```python
from build123d import *

# Parameters (mm, degrees)
SKETCH_1_R          = 100
EXTRUDE_2_DEPTH     = 50
SHELL_2_T           = -5
SKETCH_6_W          = 41.456951092
SKETCH_6_H          = 6.735302979
CUT_EXTRUDE_1_DEPTH = 10
SKETCH_9_R          = 97
CUT_EXTRUDE_2_DEPTH = 10
SKETCH_13_W         = 6
SKETCH_13_H         = 15.793483952
SKETCH_13_H_2       = 15
CUT_EXTRUDE_3_DEPTH = 10
SKETCH_16_W         = 8.245924623
SKETCH_16_H         = 19.966088532
SKETCH_16_H_2       = 20.04266097
CUT_EXTRUDE_6_DEPTH = 10
SKETCH_17_W         = 4.583098869
SKETCH_17_H         = 14.94320697
SKETCH_17_H_2       = 15.359126099
CUT_EXTRUDE_7_DEPTH = 10
SKETCH_18_W         = 6.507967363
SKETCH_18_H         = 16.40128849
SKETCH_18_H_2       = 16.311833417
CUT_EXTRUDE_8_DEPTH = 10


with BuildPart() as part:
    # Sketch 1 → Extrude 2 (new body)
    with BuildSketch(Plane.XY):
        Circle(SKETCH_1_R)
    extrude(amount=EXTRUDE_2_DEPTH)

    # Shell 2
    shell_2_openings = [part.faces().sort_by_distance(p)[0] for p in [
        (0, 0, 50),
    ]]
    offset(amount=SHELL_2_T, openings=shell_2_openings, kind=Kind.INTERSECTION)

    # Sketch 6 → Cut-Extrude 1 (cut)
    with BuildSketch(Plane.XY):
        with Locations((-20.728475546, 53.011479478)):
            Rectangle(SKETCH_6_W, SKETCH_6_H)
        with Locations((20.728475546, 53.011479478)):
            Rectangle(SKETCH_6_W, SKETCH_6_H)
    extrude(amount=CUT_EXTRUDE_1_DEPTH, mode=Mode.SUBTRACT)

    # Sketch 9 → Cut-Extrude 2 (cut)
    with BuildSketch(Plane.XY.offset(50)):
        Circle(SKETCH_9_R)
    extrude(amount=-CUT_EXTRUDE_2_DEPTH, mode=Mode.SUBTRACT)

    # Sketch 13 → Cut-Extrude 3 (cut)
    with BuildSketch(Plane.ZY.offset(100)):
        with Locations((49.635646507, 7.103258024)):
            Rectangle(SKETCH_13_W, SKETCH_13_H)
        with Locations((49.635646507, -8.293483952)):
            Rectangle(SKETCH_13_W, SKETCH_13_H_2)
    extrude(amount=-CUT_EXTRUDE_3_DEPTH, mode=Mode.SUBTRACT)

    # Sketch 16 → Cut-Extrude 6 (cut)
    with BuildSketch(Plane(origin=(100, 0, 0), x_dir=(0, 0, -1), z_dir=(1, 0, 0))):
        with Locations((-10.841517517, 9.983044266)):
            Rectangle(SKETCH_16_W, SKETCH_16_H)
        with Locations((-10.841517517, -10.021330485)):
            Rectangle(SKETCH_16_W, SKETCH_16_H_2)
    extrude(amount=-CUT_EXTRUDE_6_DEPTH, mode=Mode.SUBTRACT)

    # Sketch 17 → Cut-Extrude 7 (cut)
    with BuildSketch(Plane(origin=(-70.710678119, -70.710678119, 0), x_dir=(0, 0, -1), z_dir=(-0.7071067811865464, -0.7071067811865488, 0))):
        with Locations((-47.581138772, 7.471603485)):
            Rectangle(SKETCH_17_W, SKETCH_17_H)
        with Locations((-47.581138772, -7.67956305)):
            Rectangle(SKETCH_17_W, SKETCH_17_H_2)
    extrude(amount=-CUT_EXTRUDE_7_DEPTH, mode=Mode.SUBTRACT)

    # Sketch 18 → Cut-Extrude 8 (cut)
    with BuildSketch(Plane(origin=(-70.710678119, 70.710678119, 0), x_dir=(0, 0, 1), z_dir=(-0.7071067811865487, 0.7071067811865465, 0))):
        with Locations((49.297240538, 8.200644245)):
            Rectangle(SKETCH_18_W, SKETCH_18_H)
        with Locations((49.297240538, -8.155916709)):
            Rectangle(SKETCH_18_W, SKETCH_18_H_2)
    extrude(amount=-CUT_EXTRUDE_8_DEPTH, mode=Mode.SUBTRACT)


solid = part.part
```
Source: CAD feature listing. Evaluate the final solid. Frame: model axes, mm. A direction names the side the tool comes from. Coordinates: 2 decimals unless noted, no trailing zeros. Loops run counter-clockwise (first coordinate to the right, second up) from the corner with the lowest first, then second, coordinate; pieces in that order, holes last. Notation, with made-up numbers: (57, 21.25) - (63, 21.25) arc R19 ccw to (63, 30.25) - close; hole circle Ø11 at (67, 65.25). An arc over 180 degrees is marked (long way). Answer as CSV lines item,"result".
1. Contact query for flat-ended pins moving along their axis: pin 1 (2 mm diameter, centred on x = -98, y = -4.5, fed in from +Z); pin 2 (12 mm diameter, centred on x = 60.5, y = -67.5, fed in from +Z); pin 3 (1 mm diameter, centred on y = -57, z = 16.5, fed in from -X). Output: stop coordinate, or through.
Established:
pin 1,"stops at z = 46.64"
pin 2,"stops at z = 40"
pin 3,"stops at x = -82.51"
2. Section D-D (y = 72). Return loops of the section in (x, z), then the cut area to 3 significant figures.
Established:
outline,"(-69.4, 0) - (69.4, 0) - (69.4, 50) - (65, 50) - (65, 40) - (61.98, 40) - (61.98, 5) - (-61.98, 5) - (-61.98, 40) - (-65, 40) - (-65, 46.04) - (-69.4, 46.04) - close"
area,"1,280 mm2"
3. Section A-A (y = 0). Return loops of the section in (x, z).
Established:
outline,"(-100, 0) - (100, 0) - (100, 6.72) - (95, 6.72) - (95, 5) - (-95, 5) - (-95, 40) - (-97, 40) - (-97, 46.64) - (-100, 46.64) - close; (95, 14.96) - (100, 14.96) - (100, 50) - (97, 50) - (97, 40) - (95, 40) - close"
4. Section B-B (x = 0). Return loops of the section in (y, z).
Established:
outline,"(-100, 0) - (49.64, 0) - (49.64, 5) - (-95, 5) - (-95, 40) - (-97, 40) - (-97, 50) - (-100, 50) - close; (56.38, 0) - (100, 0) - (100, 50) - (97, 50) - (97, 40) - (95, 40) - (95, 5) - (56.38, 5) - close"
5. Ray query, line 1 (X direction, y = 0, z = 46); line 2 (X direction, y = 0, z = 16.5). Return the intervals inside material, ascending.
Established:
line 1,"x = -100 to -97, 97 to 100"
line 2,"x = -100 to -95, 95 to 100"
6. Mould query, pull axis Z, two halves, no side actions, for faces 4 (the flat face through (-1, 49.644, 2)), 5 (the flat face through (-70, -69, 45.29)), 6 (the flat face through (95, 19.966, 11)), 7 (the flat face through (71, -64, 40)). Classes: released by +Z, released by -Z, zero draft, split by the parting line, or undercut.
Established:
face 4,"zero draft"
face 5,"undercut"
face 6,"undercut"
face 7,"released by +Z"
7. Reachability of faces 1 (the flat face through (-41.457, 53, 2)), 2 (the flat face through (96, 0, 6.719)), 3 (the flat face through (-1, 1, 5)) from +Z, -Z, +X, -X, +Y, -Y: full face, straight path, thin tool, end or side. Return the list, or none.
Established:
face 1,"+Z, -Z"
face 2,"+X"
face 3,"+Z"
8. Section C-C (z = 36). Return loops of the section in (x, y).
Established:
outline,"circle Ø200 at (0, 0); hole circle Ø190 at (0, 0)"
